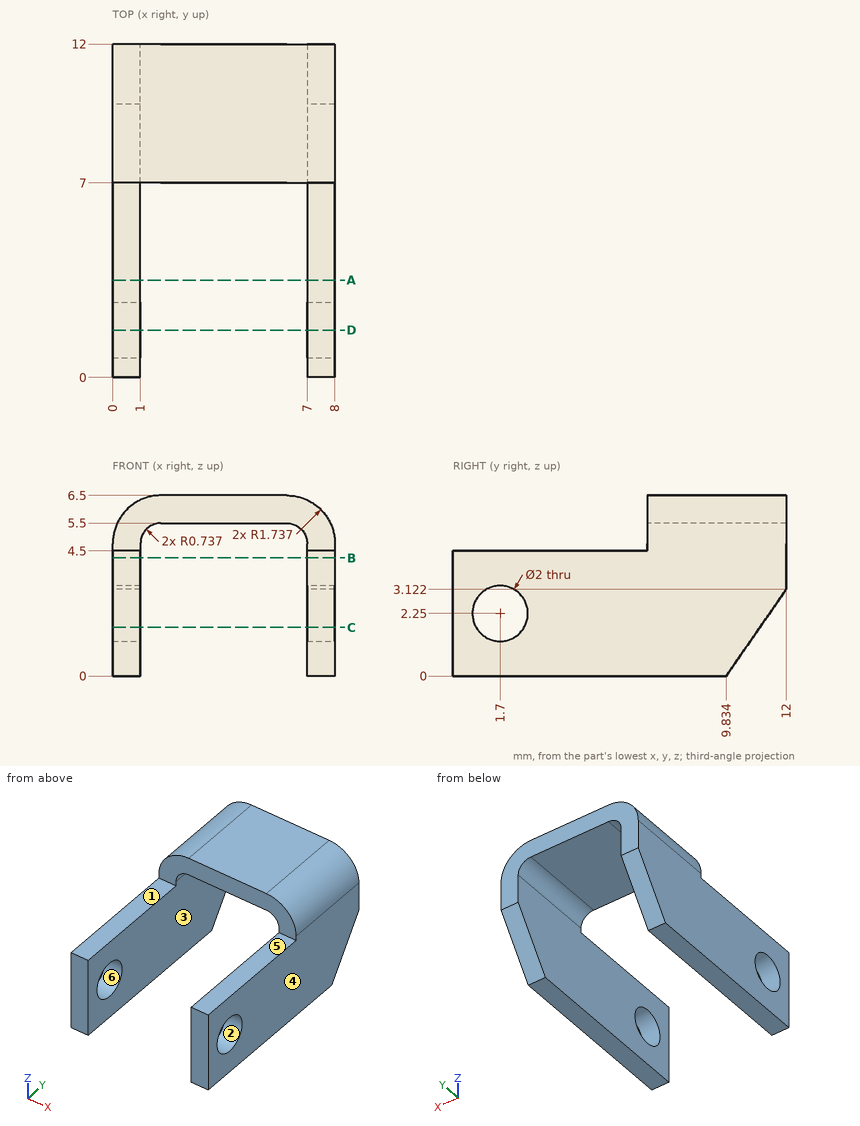
Geometry: see drawing. Coordinates: mm, zero at the bounding-box minimum. A direction names the side the tool comes from. Round coordinates to 2 decimals unless told otherwise and drop trailing zeros. Write each loop counter-clockwise with the first axis right and the second up, starting at its lowest first coordinate (ties: lowest second). Pieces come first, ordered by that corner, then holes.
Item 1: Section query A-A (y = 3.5). Return loops of the section in (x, z).
Item 2: Material intervals for L1, parallel to X at y = 8.25, z = 2.5; L2, parallel to Z at x = 0.5, y = 1.7; L3, parallel to Z at x = 4, y = 11.5, sorted ascending.
Item 3: Mould query, pull axis Z, two halves, no side actions, for the marked faces 4, 5 and 6. Classes: +Z half, -Z half, draft (parallel to the pull), parting line (faces both ways), or undercut.
Item 4: Section query C-C (z = 1.75). Return loops of the section in (x, y).
Item 5: Pin query (flat end, axial travel): P1, Ø1.4, axis at y = 8, z = 2.5, coming from the -X side; P2, Ø1.1, axis at x = 0.5, y = 3, coming from the +Z side; P3, Ø1.4, axis at x = 4, y = 8.5, coming from the -Z side; P4, Ø1.5, axis at x = 6, z = 1, coming from the +Y side. Return the tip coordinate at first contact, or that it passes through.
Item 6: Set-up query: the marked faces 1, 2 and 3. Return all of +Z, -Z, +X, -X, +Y, -Y with unobstructed straight access to the full face (end or side cutting, diameter ignored); none if empty.
Item 7: Section query B-B (z = 4.25). Return loops of the section in (x, y), plus the area to 3 significant figures.
Item 8: Section query D-D (y = 1.7). Return loops of the section in (x, z).
Completed:
1. outline: (0, 0) - (1, 0) - (1, 4.5) - (0, 4.5) - close; (7, 0) - (8, 0) - (8, 4.5) - (7, 4.5) - close
2. L1: x = 0 to 1, 7 to 8
2. L2: z = 0 to 1.25, 3.25 to 4.5
2. L3: z = 5.5 to 6.5
3. face 4: draft
3. face 5: +Z half
3. face 6: undercut
4. outline: (0, 0) - (1, 0) - (1, 0.83) - (0, 0.83) - close; (0, 2.57) - (1, 2.57) - (1, 11.05) - (0, 11.05) - close; (7, 0) - (8, 0) - (8, 0.83) - (7, 0.83) - close; (7, 2.57) - (8, 2.57) - (8, 11.05) - (7, 11.05) - close
5. P1: stops at x = 0
5. P2: stops at z = 4.5
5. P3: stops at z = 5.5
5. P4: passes through
6. face 1: +Z, +X, -X, -Y
6. face 2: +X, -X
6. face 3: -Z, +Y, -Y
7. outline: (0, 0) - (1, 0) - (1, 12) - (0, 12) - close; (7, 0) - (8, 0) - (8, 12) - (7, 12) - close
7. area: 24.0 mm2
8. outline: (0, 0) - (1, 0) - (1, 1.25) - (0, 1.25) - close; (0, 3.25) - (1, 3.25) - (1, 4.5) - (0, 4.5) - close; (7, 0) - (8, 0) - (8, 1.25) - (7, 1.25) - close; (7, 3.25) - (8, 3.25) - (8, 4.5) - (7, 4.5) - close
